The drawing under review shows one solid part. Ordinate dimensions are in mm from its lowest x, y, z. A direction names the side the tool comes from. Give positions to 0.01 mm unless a question says otherwise; leave off trailing zeros. Loops run counter-clockwise (first coordinate to the right, second up) from the corner with the lowest first, then second, coordinate; pieces in that order, holes last. Notation, with made-up numbers: (-13, 62.25) - (44, 62.25) arc R13 cw to (44, 66.25) - close; hole circle Ø10 at (39, 64.25). An arc over 180 degrees is marked (long way). Write each question's results on one line, items separated by ' | '.
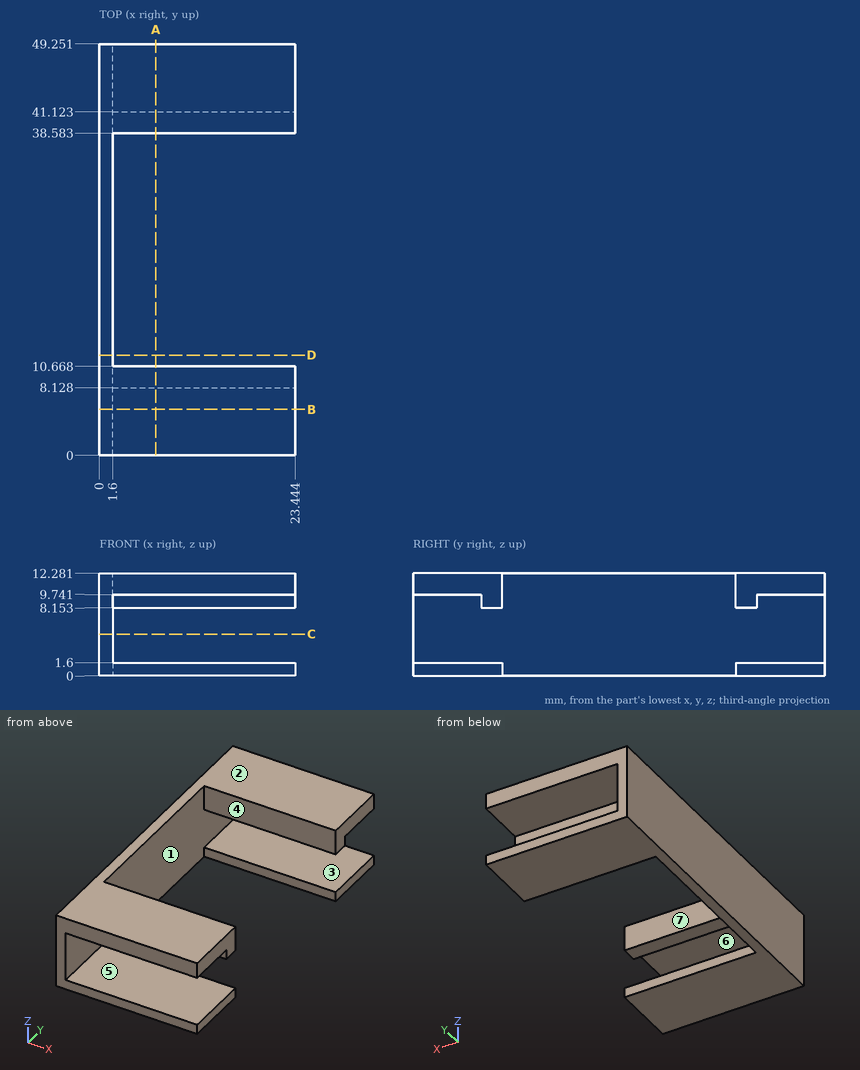
(1) Take a section at C-C on z = 5. Give the boundary of the cut face in (x, y).
Answers below:
outline: (0, 0) - (1.6, 0) - (1.6, 49.25) - (0, 49.25) - close
(2) Take a section at D-D on y = 12. Give the boundary of the cut face in (x, z).
Answers below:
outline: (0, 0) - (1.6, 0) - (1.6, 12.28) - (0, 12.28) - close
(3) Wall thickness on line 1 along Z through (x, y) = (6, 42); line 2 along Y through (x, z) = (18.5, 11.75); line 3 along Z through (x, y) = (16.5, 40.5): over which ranges is each line inside the solid? List them lowest first. Write a range as from..to.
Answers below:
line 1: 0..1.6, 9.74..12.28 | line 2: 0..10.67, 38.58..49.25 | line 3: 0..1.6, 8.15..12.28
(4) Draft analysis for pull direction Z (two halves, no side actions). For the marked faces 1, 2, 3 and 4, state which applies: pulls with the +Z half, pulls with the -Z half, needs draft (parallel to the pull), parting line crosses it, or undercut.
Answers below:
face 1: undercut | face 2: pulls with the +Z half | face 3: undercut | face 4: needs draft
(5) Take a section at B-B on y = 5.5. Give the boundary of the cut face in (x, z) (1 decimal).
Answers below:
outline: (0, 0) - (23.4, 0) - (23.4, 1.6) - (1.6, 1.6) - (1.6, 9.7) - (23.4, 9.7) - (23.4, 12.3) - (0, 12.3) - close
(6) Tool access review of the marked faces 5, 6 and 7: name each direction out of +Z, -Z, +X, -X, +Y, -Y from which nothing blocks a thin tool from reaching the whole face with its end or side.
Answers below:
face 5: +X, +Y, -Y | face 6: +X, -Y | face 7: +Z, -Z, +X
(7) Insertion check: P1, Ø0.8, axis at x = 13, z = 9, coming from the -Y side; P2, Ø6, axis at y = 16.5, z = 4.5, coming from the +X side; P3, Ø0.5, axis at x = 7, z = 9, coming from the +Y side. Each pin has a flat end and moves straight along its axis. Give the tip position at first contact, or say it passes through.
Answers below:
P1: y = 8.13 | P2: x = 1.6 | P3: y = 41.12
(8) Take a section at A-A on x = 6.75. Give the boundary of the cut face in (y, z).
Answers below:
outline: (0, 0) - (10.67, 0) - (10.67, 1.6) - (0, 1.6) - close; (0, 9.74) - (8.13, 9.74) - (8.13, 8.15) - (10.67, 8.15) - (10.67, 12.28) - (0, 12.28) - close; (38.58, 0) - (49.25, 0) - (49.25, 1.6) - (38.58, 1.6) - close; (38.58, 8.15) - (41.12, 8.15) - (41.12, 9.74) - (49.25, 9.74) - (49.25, 12.28) - (38.58, 12.28) - close
